Autodesk Inventor part; units mm, degrees
ref_plane "YZ Plane" through (0, 0, 0) normal (1, 0, 0) x (0, 1, 0)
ref_plane "XZ Plane" through (0, 0, 0) normal (0, 1, 0) x (-1, 0, 0)
ref_plane "XY Plane" through (0, 0, 0) normal (0, 0, 1) x (1, 0, 0)
sketch "Sketch1" plane through (0, 0, 0) normal (0, 0, 1) x (1, 0, 0)
  line L0 (0, 0) -> (-4, 0)
  line L1 (-4, 0) -> (-4, 10)
  line L2 (-4, 10) -> (0, 10)
  line L3 (0, 10) -> (0, 0)
  line L4 (-28, 0) -> (-24, 0)
  line L5 (-24, 0) -> (-24, 10)
  line L6 (-24, 10) -> (-28, 10)
  line L7 (-28, 10) -> (-28, 0)
  dimension "d0" = 4
  dimension "d1" = 10
extrude "Extrusion1" add sketch "Sketch1" along normal blind 1950
sketch "Sketch2" plane through (0, 0, 1950) normal (0, 0, 1) x (1, 0, 0)
  line L0 (-24, 10) -> (-28, 10)
  line L1 (-28, 10) -> (0, 10)
  line L2 (0, 10) -> (0, 0)
  line L3 (0, 0) -> (-28, 0)
  line L4 (-28, 0) -> (-28, 10)
extrude "Extrusion2" add sketch "Sketch2" along normal blind 10
sketch "Sketch3" plane through (0, 0, 0) normal (0, 0, -1) x (-1, 0, 0)
  line L0 (0, 0) -> (4, 0)
  line L1 (0, 0) -> (28, 0)
  line L2 (28, 0) -> (28, 10)
  line L3 (28, 10) -> (0, 10)
  line L4 (0, 10) -> (0, 0)
extrude "Extrusion3" add sketch "Sketch3" along normal blind 10
Work out the finished part from the listing and answer in its coordinate system (mm). Coordinates: 2 decimals unless noted, no trailing zeros. Write each loop counter-clockwise with the first axis right and the second up, starting at its lowest first coordinate (ties: lowest second). Pieces come first, ordered by that corner, then holes. Notation, with made-up numbers: M 19.25,30 L 42.25,30 A14 cw 42.25,43 Z; hole C 53,39.25 d10. An arc over 180 degrees is marked long. Write item = value, one per line.
1. Straight lines are drawn through the part: line 1 (Z direction, x = -19, y = 2.5); line 2 (X direction, y = 6.75, z = 1618). For each, find the intervals that lie inside material, in ascending order. Write a range as from..to.
Solution:
line_1 = -10..0, 1950..1960
line_2 = -28..-24, -4..0
2. The part is cut by section B-B (x = -14.5). Determine the outline of the cut face in (y, z).
Solution:
outline = M 0,-10 L 10,-10 L 10,0 L 0,0 Z; M 0,1950 L 10,1950 L 10,1960 L 0,1960 Z
3. The part is cut by section A-A (z = 1379). Determine the outline of the cut face in (x, y), then the cut area to 3 significant figures.
Solution:
outline = M -28,0 L -24,0 L -24,10 L -28,10 Z; M -4,0 L 0,0 L 0,10 L -4,10 Z
area = 80.0 mm2
4. The part is cut by section C-C (y = 1.75). Determine the outline of the cut face in (x, z).
Solution:
outline = M -28,-10 L 0,-10 L 0,1960 L -28,1960 Z; hole M -24,0 L -4,0 L -4,1950 L -24,1950 Z
